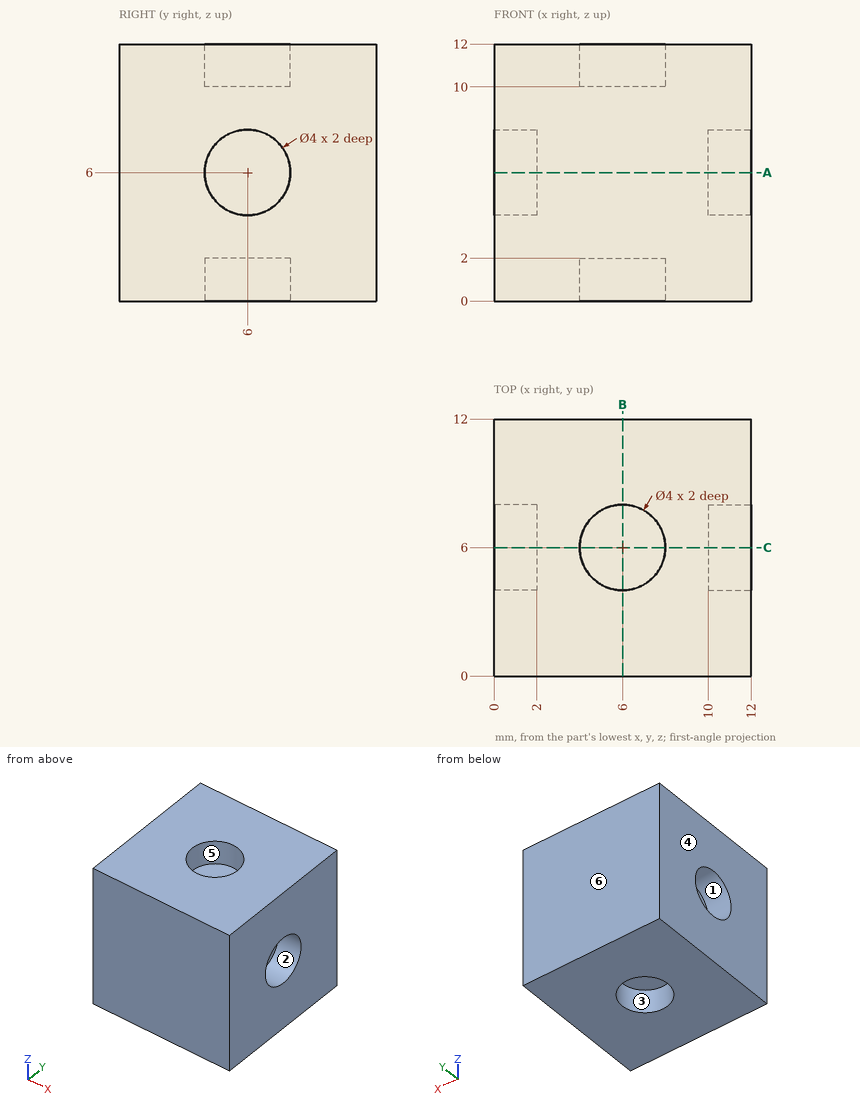
Source: three-view drawing plus pictorial views. Frame: mm from the lowest corner of the part. A direction names the side the tool comes from. Coordinates: 2 decimals unless noted, no trailing zeros. Write each loop counter-clockwise with the first axis right and the second up, starting at its lowest first coordinate (ties: lowest second). Pieces come first, ordered by that corner, then holes. Notation, with made-up numbers: (29.25, 42.25) - (72.25, 42.25) arc R15 cw to (72.25, 70.25) - close; hole circle Ø6 at (25, 11). An arc over 180 degrees is marked (long way). Return JSON: item names as keys, results as strings.
Item 1: Reachability of the marked faces 1, 2 and 3 from +Z, -Z, +X, -X, +Y, -Y: full face, straight path, thin tool, end or side. Return the list, or none.
Completed:
{"face 1": "-X", "face 2": "+X", "face 3": "-Z"}
Item 2: Section query A-A (z = 6). Output: boundary loops of the cut face in (x, y).
Completed:
{"outline": "(0, 0) - (12, 0) - (12, 4) - (10, 4) - (10, 8) - (12, 8) - (12, 12) - (0, 12) - (0, 8) - (2, 8) - (2, 4) - (0, 4) - close"}
Item 3: Pin query (flat end, axial travel): pin 1 Ø3.5 at (y, z) = (6, 6) entering from +X; pin 2 Ø1.2 at (x, y) = (5.5, 6) entering from +Z; pin 3 Ø1.2 at (y, z) = (6.5, 5) entering from -X. Return the tip coordinate at first contact, or that it passes through.
Completed:
{"pin 1": "stops at x = 10", "pin 2": "stops at z = 10", "pin 3": "stops at x = 2"}
Item 4: Section query B-B (x = 6). Output: boundary loops of the cut face in (y, z), and give its area (3 significant figures).
Completed:
{"outline": "(0, 0) - (4, 0) - (4, 2) - (8, 2) - (8, 0) - (12, 0) - (12, 12) - (8, 12) - (8, 10) - (4, 10) - (4, 12) - (0, 12) - close", "area": "128 mm2"}
Item 5: Line query: L1, parallel to Y at x = 6, z = 1; L2, parallel to Z at x = 5.25, y = 4.75. Output: solid intervals per line, ascending.
Completed:
{"L1": "y = 0 to 4, 8 to 12", "L2": "z = 2 to 10"}
Item 6: Pull-direction query (X, two-part tool) for the marked faces 4, 5 and 6; classes: +X half, -X half, draft (parallel to the pull), parting line (faces both ways), or undercut.
Completed:
{"face 4": "-X half", "face 5": "undercut", "face 6": "draft"}
Item 7: Section query C-C (y = 6). Output: boundary loops of the cut face in (x, z), and give its area (3 significant figures).
Completed:
{"outline": "(0, 0) - (4, 0) - (4, 2) - (8, 2) - (8, 0) - (12, 0) - (12, 4) - (10, 4) - (10, 8) - (12, 8) - (12, 12) - (8, 12) - (8, 10) - (4, 10) - (4, 12) - (0, 12) - (0, 8) - (2, 8) - (2, 4) - (0, 4) - close", "area": "112 mm2"}
